Geometry check sheet. Reference: the model listing, model coordinates, mm. Face numbers are marked on the shaded views. A direction names the side the tool comes from. Coordinates: 2 decimals unless noted, no trailing zeros. Order: outer loops, then holes, each group sorted by start corner. A loop starts at its lowest first (then second) coordinate and runs counter-clockwise, first axis right, second up. Notation, with made-up numbers: (31, 50.25) -> (77, 50.25) arc R12 cw to (77, 62.25) -> close; hole circle Ø9 at (-27.5, 46.5). An arc over 180 degrees is marked (long way). Answer in a Markdown table with one row per item. Add a question column.
```python
from build123d import *

# Parameters (mm, degrees)
EXTRUDE_1_DEPTH     = 3
SKETCH_2_W          = 156
SKETCH_2_H          = 45
EXTRUDE_2_DEPTH     = 3
SKETCH_3_R          = 1.5
CUT_EXTRUDE_1_DEPTH = 3
SKETCH_4_W          = 130
SKETCH_4_H          = 20
CUT_EXTRUDE_2_DEPTH = 3
FILLET_1_R          = 10
CHAMFER_1_SIZE      = 0.5
FILLET_2_R          = 10
CHAMFER_2_SIZE      = 0.5


with BuildPart() as part:
    # 草图1 → 凸台-拉伸1 (new body)
    with BuildSketch(Plane.XY):
        with BuildLine():
            Line((-120, -15), (120, -15))
            Line((120, -15), (120, -90.328663107))
            ThreePointArc((120, -90.328663107), (0, -125), (-120, -90.328663107))
            Line((-120, -90.328663107), (-120, -15))
        make_face()
    extrude(amount=EXTRUDE_1_DEPTH)

    # 草图2 → 凸台-拉伸2 (add)
    with BuildSketch(Plane.XY.offset(3)):
        with Locations((0, -37.5)):
            Rectangle(SKETCH_2_W, SKETCH_2_H)
    extrude(amount=EXTRUDE_2_DEPTH)

    # 草图3 → 切除-拉伸1 (cut)
    with BuildSketch(Plane(origin=(0, 0, 0), x_dir=(-1, 0, 0), z_dir=(0, 0, -1))):
        with Locations((30, -100)):
            Circle(SKETCH_3_R)
        with Locations((113, -45)):
            Circle(SKETCH_3_R)
        with Locations(Location((-113, -45, 0), (0, 0, 180))):
            Circle(SKETCH_3_R)
        with Locations(Location((-30, -100, 0), (0, 0, 180))):
            Circle(SKETCH_3_R)
    extrude(amount=-CUT_EXTRUDE_1_DEPTH, mode=Mode.SUBTRACT)

    # 草图4 → 切除-拉伸2 (cut)
    with BuildSketch(Plane(origin=(0, 0, 0), x_dir=(-1, 0, 0), z_dir=(0, 0, -1))):
        with Locations((0, -25)):
            Rectangle(SKETCH_4_W, SKETCH_4_H)
    extrude(amount=-CUT_EXTRUDE_2_DEPTH, mode=Mode.SUBTRACT)

    # 圆角1
    fillet_1_edges = [part.edges().sort_by_distance(p)[0] for p in [
        (120, -90.328663107, 1.5),
        (-120, -90.328663107, 1.5),
    ]]
    fillet(fillet_1_edges, radius=FILLET_1_R)

    # 倒角1
    chamfer_1_edges = [part.edges().sort_by_distance(p)[0] for p in [
        (-92.5, -15, 0),
        (92.5, -15, 0),
        (65, -25, 0),
        (0, -35, 0),
        (-65, -25, 0),
    ]]
    chamfer(chamfer_1_edges, length=CHAMFER_1_SIZE)

    # 圆角2
    fillet_2_edges = [part.edges().sort_by_distance(p)[0] for p in [
        (-78, -60, 4.5),
        (78, -60, 4.5),
    ]]
    fillet(fillet_2_edges, radius=FILLET_2_R)

    # 倒角2
    chamfer_2_edges = [part.edges().sort_by_distance(p)[0] for p in [
        (-75.071067812, -57.071067812, 6),
        (-78, -32.5, 6),
        (0, -60, 6),
        (78, -32.5, 6),
        (75.071067812, -57.071067812, 6),
    ]]
    chamfer(chamfer_2_edges, length=CHAMFER_2_SIZE)


solid = part.part
```
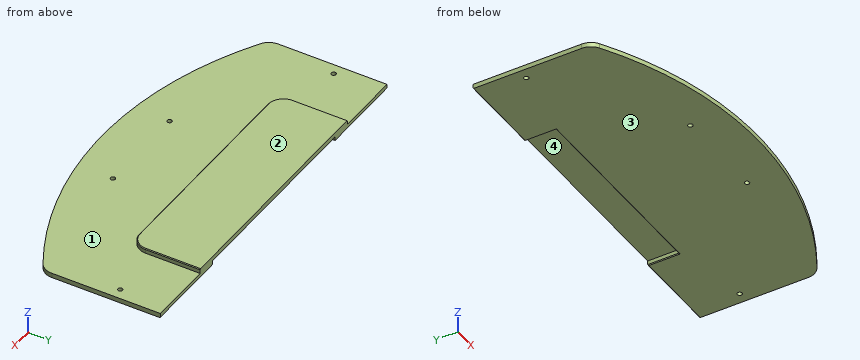
(1) Mould release check, pull along X, two halves, no side actions. Record for the marked faces 3 and 4: +X half, -X half, draft (parallel to the pull), parting line (faces both ways), or undercut.
(2) Cross-section at D-D (y = -68). Enter the section's corners in (x, z).
(3) Cross-section at A-A (z = 2). Enter the section's corners in (x, y).
(4) Cross-section at B-B (y = -27.5). Enter the section's corners in (x, z).
(5) Cross-section at C-C (x = 61.5). Enter the section's corners in (y, z), plus the area to 3 significant figures.
(6) Scan lines: line 1 along X through (y, z) = (-100, 0.65); line 2 along Z through (x, y) = (-3, -101.5); line 3 along Z through (x, y) = (9, -25). Record each from-to range of solid material in increasing order.
(7) Go/stop test with flat-tipped pins: P1, Ø3.5, axis at x = -30, y = -100, coming from the +Z side; P2, Ø2, axis at x = -18.5, z = 1.5, coming from the +Y side; P3, Ø1.5, axis at x = -61.5, y = -60.5, coming from the +Z side; P4, Ø2.5, axis at x = 30, y = -100, coming from the +Z side. Record where each tip stops, or that it passes through.
(8) Access from +Z, -Z, +X, -X, +Y, -Y to the whole of each face (thin tool, end or side, straight path). Record for the marked faces 1 and 2.
Checks:
| question | item | result |
|---|---|---|
| 1 | face 3 | draft |
| 1 | face 4 | undercut |
| 2 | outline | (-120, 0) -> (120, 0) -> (120, 3) -> (-120, 3) -> close |
| 3 | outline | (-120, -84.73) arc R10 ccw to (-115.12, -93.32) arc R225 ccw to (115.12, -93.32) arc R10 ccw to (120, -84.73) -> (120, -15) -> (65, -15) -> (65, -35) -> (-65, -35) -> (-65, -15) -> (-120, -15) -> close; hole circle Ø3 at (-113, -45); hole circle Ø3 at (-30, -100); hole circle Ø3 at (30, -100); hole circle Ø3 at (113, -45) |
| 4 | outline | (-120, 0) -> (-65.5, 0) -> (-65, 0.5) -> (-65, 3) -> (65, 3) -> (65, 0.5) -> (65.5, 0) -> (120, 0) -> (120, 3) -> (78, 3) -> (78, 5.5) -> (77.5, 6) -> (-77.5, 6) -> (-78, 5.5) -> (-78, 3) -> (-120, 3) -> close |
| 5 | outline | (-116.43, 0) -> (-35.5, 0) -> (-35, 0.5) -> (-35, 3) -> (-15, 3) -> (-15, 6) -> (-59.5, 6) -> (-60, 5.5) -> (-60, 3) -> (-116.43, 3) -> close |
| 5 | area | 379 mm² |
| 6 | line 1 | -103.08 to -31.5, -28.5 to 28.5, 31.5 to 103.08 |
| 6 | line 2 | 0 to 3 |
| 6 | line 3 | 3 to 6 |
| 7 | P1 | z = 3 |
| 7 | P2 | y = -35 |
| 7 | P3 | z = 5.75 |
| 7 | P4 | through |
| 8 | face 1 | +Z, -Y |
| 8 | face 2 | +Z, +X, -X, +Y, -Y |
